```python
from build123d import *

# Parameters (mm, degrees)
CROQUIS1_W                 = 40
CROQUIS1_H                 = 65
CROQUIS1_R                 = 10
SALIENTE_EXTRUIR1_DEPTH    = 40
CROQUIS2_W                 = 60
CROQUIS2_H                 = 55
CORTAR_EXTRUIR1_DEPTH      = 21
CORTAR_EXTRUIR1_DEPTH_BACK = 21
CROQUIS3_W                 = 20
CROQUIS3_H                 = 5
CORTAR_EXTRUIR2_DEPTH      = 41
CORTAR_EXTRUIR2_DEPTH_BACK = 41


with BuildPart() as part:
    # Croquis1 → Saliente-Extruir1 (new body, symmetric)
    with BuildSketch(Plane(origin=(0, 0, 0), x_dir=(0, 0, -1), z_dir=(1, 0, 0))):
        with Locations((0, 17.5)):
            Rectangle(CROQUIS1_W, CROQUIS1_H)
        Circle(CROQUIS1_R, mode=Mode.SUBTRACT)
    extrude(amount=SALIENTE_EXTRUIR1_DEPTH, both=True)

    # Croquis2 → Cortar-Extruir1 (cut, two sides)
    with BuildSketch(Plane.XY) as cortar_extruir1_sk:
        with Locations((0, 12.5)):
            Rectangle(CROQUIS2_W, CROQUIS2_H)
    extrude(amount=CORTAR_EXTRUIR1_DEPTH, mode=Mode.SUBTRACT)
    extrude(cortar_extruir1_sk.sketch, amount=-CORTAR_EXTRUIR1_DEPTH_BACK, mode=Mode.SUBTRACT)

    # Croquis3 → Cortar-Extruir2 (cut, two sides)
    with BuildSketch(Plane(origin=(0, 0, 0), x_dir=(0, 0, -1), z_dir=(1, 0, 0))) as cortar_extruir2_sk:
        with Locations((10, 47.5)):
            Rectangle(CROQUIS3_W, CROQUIS3_H)
    extrude(amount=CORTAR_EXTRUIR2_DEPTH, mode=Mode.SUBTRACT)
    extrude(cortar_extruir2_sk.sketch, amount=-CORTAR_EXTRUIR2_DEPTH_BACK, mode=Mode.SUBTRACT)


solid = part.part
```
The model under review builds one solid part; all positions refer to its coordinate system, in mm. A direction names the side the tool comes from. Round coordinates to 2 decimals unless told otherwise and drop trailing zeros. Loops run counter-clockwise (first coordinate to the right, second up) from the corner with the lowest first, then second, coordinate; pieces in that order, holes last.
1) Consider section C-C on y = 0. State the section outline as (x, z) points.
Values follow:
outline: (-40, -20) - (-30, -20) - (-30, -10) - (-40, -10) - close; (-40, 10) - (-30, 10) - (-30, 20) - (-40, 20) - close; (30, -20) - (40, -20) - (40, -10) - (30, -10) - close; (30, 10) - (40, 10) - (40, 20) - (30, 20) - close
2) Tool access review of faces 1 (the face through (-1, 47, 0)), 2 (the face through (0, 41, 20)), 3 (the face through (-30, 12, 0)): name each direction out of +Z, -Z, +X, -X, +Y, -Y from which nothing blocks a thin tool from reaching the whole face with its end or side.
Values follow:
face 1: -Z, +X, -X, +Y
face 2: +Z, +X, -X, +Y, -Y
face 3: +Z, -Z, -Y
3) Consider section A-A on y = 12. State the section outline as (x, z) points, then the cut area to 3 significant figures.
Values follow:
outline: (-40, -20) - (-30, -20) - (-30, 20) - (-40, 20) - close; (30, -20) - (40, -20) - (40, 20) - (30, 20) - close
area: 800 mm2
4) The part is to be moulded in two halves that separate along X. For faces 4 (the face through (0, 40, 0)), 5 (the face through (-40, 18, 0)), 6 (the face through (40, 18, 0)), 7 (the face through (-35.07, -9.76, 2.17)), say which applies: pulls with the +X half, pulls with the -X half, needs draft (parallel to the pull), parting line crosses it, or undercut.
Values follow:
face 4: undercut
face 5: pulls with the -X half
face 6: pulls with the +X half
face 7: needs draft
5) Consider section B-B on z = 8. State the section outline as (x, y) points, then the cut area to 3 significant figures.
Values follow:
outline: (-40, -15) - (-30, -15) - (-30, -6) - (-40, -6) - close; (-40, 6) - (-30, 6) - (-30, 40) - (30, 40) - (30, 6) - (40, 6) - (40, 50) - (-40, 50) - close; (30, -15) - (40, -15) - (40, -6) - (30, -6) - close
area: 1,660 mm2
6) Consider section D-D on z = 12. State the section outline as (x, y) points, then the cut area to 3 significant figures.
Values follow:
outline: (-40, -15) - (-30, -15) - (-30, 40) - (30, 40) - (30, -15) - (40, -15) - (40, 50) - (-40, 50) - close
area: 1,900 mm2
7) Clearance check with flat-ended pins moving along their axes: P1, Ø10, axis at x = 0.5, z = -2, coming from the -Y side; P2, Ø3, axis at x = -20, z = -11.5, coming from the +Y side; P3, Ø4, axis at x = -15.5, y = 47.5, coming from the -Z side. State where each tip first meets the part, or that it passes through.
Values follow:
P1: stops at y = 40
P2: stops at y = 45
P3: stops at z = 0
8) Wall thickness on line 1 along Z through (x, y) = (-34, 0); line 2 along X through (y, z) = (-11, -8); line 3 along Y through (x, z) = (-28.5, 15.5): over which ranges is each line inside the solid? List them lowest first.
Values follow:
line 1: z = -20 to -10, 10 to 20
line 2: x = -40 to -30, 30 to 40
line 3: y = 40 to 50
